Here's how the part is built. I have some questions about the finished solid (model axes, mm). Coordinates: 2 decimals unless noted, no trailing zeros. Order: outer loops, then holes, each group sorted by start corner. A loop starts at its lowest first (then second) coordinate and runs counter-clockwise, first axis right, second up. Notation, with made-up numbers: (86.5, 42.5) -> (136.5, 42.5) arc R27 ccw to (136.5, 68.5) -> close; hole circle Ø8 at (63, 75.25). An arc over 180 degrees is marked (long way). One line per item, written item: value. Start each with the question number.
Autodesk Inventor part; units mm, degrees
ref_plane "YZ Plane" through (0, 0, 0) normal (1, 0, 0) x (0, 1, 0)
ref_plane "XZ Plane" through (0, 0, 0) normal (0, 1, 0) x (-1, 0, 0)
ref_plane "XY Plane" through (0, 0, 0) normal (0, 0, 1) x (1, 0, 0)
sketch "Sketch1" plane through (0, 0, 0) normal (0, 0, 1) x (1, 0, 0)
  circle A0 centre (0, 0) radius 10.5
  line L0 (0, 0) -> (8, 0)
  circle A1 centre (8, 0) radius 1.25
  circle A2 centre (5.6569, 5.6569) radius 1.25
  circle A3 centre (0, 8) radius 1.25
  circle A4 centre (-5.6569, 5.6569) radius 1.25
  circle A5 centre (-8, 0) radius 1.25
  circle A6 centre (-5.6569, -5.6569) radius 1.25
  circle A7 centre (0, -8) radius 1.25
  circle A8 centre (5.6569, -5.6569) radius 1.25
  dimension "d0" = 21
  dimension "d1" = 8
  dimension "d2" = 2.5
  dimension "d5" = 360
extrude "Extrusion1" add sketch "Sketch1" along normal blind 6
sketch "Sketch2" plane through (0, 0, 6) normal (0, 0, 1) x (1, 0, 0)
  circle A0 centre (0, 0) radius 4.5
  dimension "d9" = 9
extrude "Extrusion2" cut sketch "Sketch2" against normal blind 6
properties part number "Motor_horn_mount"
Q1. Imagine slicing it at A-A (x = 0). Write out the boundary of the cut face in (y, z).
Q2. Imagine slicing it at D-D (y = 2.5). Write out the boundary of the cut face in (x, z).
Q3. Imagine slicing it at C-C (x = -8). Write out the boundary of the cut face in (y, z), plus the area to 3 significant figures.
Q4. I need wall thicknesses on line 1 (Y direction, x = 0, z = 2.75); line 2 (Y direction, x = 6.25, z = 3.05); line 3 (Y direction, x = -5.25, z = 3.9). Which ranges of each line are inside material? Lowest first, please.
Q5. If we mould it in two halves opening along X, with no side actions, what happens to faces 1 (the face through (5, 0, 0)), 2 (the face through (10, -3.2, 3)), 3 (the face through (-0.27, -6.78, 2.96))? For each: +X half, -X half, draft (parallel to the pull), parting line (faces both ways), or undercut.
Completed:
1. outline: (-10.5, 0) -> (-9.25, 0) -> (-9.25, 6) -> (-10.5, 6) -> close; (-6.75, 0) -> (-4.5, 0) -> (-4.5, 6) -> (-6.75, 6) -> close; (4.5, 0) -> (6.75, 0) -> (6.75, 6) -> (4.5, 6) -> close; (9.25, 0) -> (10.5, 0) -> (10.5, 6) -> (9.25, 6) -> close
2. outline: (-10.2, 0) -> (-3.74, 0) -> (-3.74, 6) -> (-10.2, 6) -> close; (3.74, 0) -> (10.2, 0) -> (10.2, 6) -> (3.74, 6) -> close
3. outline: (-6.8, 0) -> (-1.25, 0) -> (-1.25, 6) -> (-6.8, 6) -> close; (1.25, 0) -> (6.8, 0) -> (6.8, 6) -> (1.25, 6) -> close
3. area: 66.6 mm2
4. line 1: y = -10.5 to -9.25, -6.75 to -4.5, 4.5 to 6.75, 9.25 to 10.5
4. line 2: y = -8.44 to -6.76, -4.56 to 4.56, 6.76 to 8.44
4. line 3: y = -9.09 to -6.84, -4.47 to 4.47, 6.84 to 9.09
5. face 1: draft
5. face 2: parting line
5. face 3: undercut
